```python
from build123d import *

# Parameters (mm, degrees)
BASE_FLANGE1_DEPTH = 2.3
TAB1_DEPTH         = 2.3


# Sheet-metal steps are written as plain solids
with BuildPart() as part:
    # Sketch1 → Base-Flange1 (new body)
    with BuildSketch(Plane(origin=(0, 0, 0), x_dir=(1, 0, 0), z_dir=(0, 1, 0))):
        with BuildLine():
            Line((-1, -2.15), (-2, -2.15))
            ThreePointArc((-2, -2.15), (-2.707106781, -1.857106781), (-3, -1.15))
            Line((-3, -1.15), (-3, 3.15))
            ThreePointArc((-3, 3.15), (-2.707106781, 3.857106781), (-2, 4.15))
            Line((-2, 4.15), (2, 4.15))
            ThreePointArc((2, 4.15), (2.707106781, 3.857106781), (3, 3.15))
            Line((3, 3.15), (3, -1.15))
            ThreePointArc((3, -1.15), (2.707106781, -1.857106781), (2, -2.15))
            Line((2, -2.15), (1, -2.15))
            Line((1, -2.15), (1, 2.15))
            Line((1, 2.15), (-1, 2.15))
            Line((-1, 2.15), (-1, -2.15))
        make_face()
    extrude(amount=-BASE_FLANGE1_DEPTH)

    # Sketch6 → Tab1 (add)
    with BuildSketch(Plane(origin=(0, 0, 0), x_dir=(1, 0, 0), z_dir=(0, 1, 0))):
        with BuildLine():
            Line((-1, -1.9), (-1, -1.4))
            ThreePointArc((-1, -1.4), (-0.75, -1.65), (-1, -1.9))
        make_face()
        with BuildLine():
            Line((1, -1.9), (1, -1.4))
            ThreePointArc((1, -1.4), (0.75, -1.65), (1, -1.9))
        make_face()
    extrude(amount=-TAB1_DEPTH)


solid = part.part
```
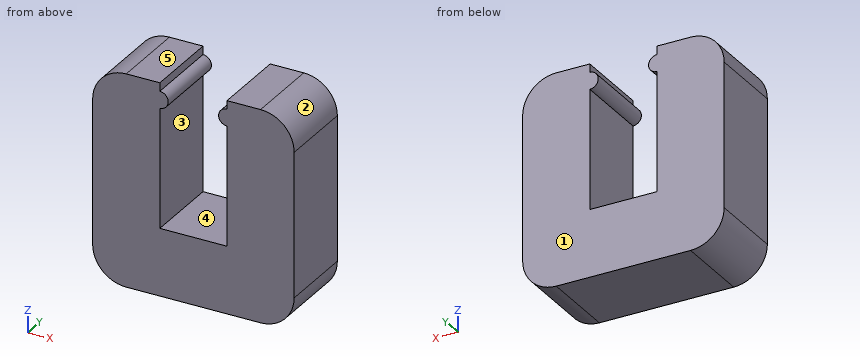
Source: CAD feature listing. Evaluate the final solid. Frame: model axes, mm. Face numbers are marked on the shaded views. A direction names the side the tool comes from. Coordinates: 2 decimals unless noted, no trailing zeros. Order: outer loops, then holes, each group sorted by start corner. A loop starts at its lowest first (then second) coordinate and runs counter-clockwise, first axis right, second up. Notation, with made-up numbers: (6, 86) - (60, 86) arc R12 ccw to (60, 102) - close; hole circle Ø6 at (-28, 14.5). An arc over 180 degrees is marked (long way). One line per item, written item: value.
1) Cut plane A-A on z = 0.5. Output: boundary loops of the cut face in (x, y), plus the area to 3 significant figures.
Computed values:
outline: (-3, -2.3) - (-1, -2.3) - (-1, 0) - (-3, 0) - close; (1, -2.3) - (3, -2.3) - (3, 0) - (1, 0) - close
area: 9.20 mm^2
2) Reachability of the marked faces 4 and 5 from +Z, -Z, +X, -X, +Y, -Y: full face, straight path, thin tool, end or side. Return the list, or none.
Computed values:
face 4: +Y, -Y
face 5: +Z, +X, -X, +Y, -Y
3) Cut plane D-D on x = -2.5. Output: boundary loops of the cut face in (y, z).
Computed values:
outline: (-2.3, -4.02) - (0, -4.02) - (0, 2.02) - (-2.3, 2.02) - close
4) Cut plane C-C on z = 1.65. Output: boundary loops of the cut face in (x, y).
Computed values:
outline: (-2.87, -2.3) - (-0.75, -2.3) - (-0.75, 0) - (-2.87, 0) - close; (0.75, -2.3) - (2.87, -2.3) - (2.87, 0) - (0.75, 0) - close
5) Ray query, line 1 (X direction, y = -1.35, z = 0); line 2 (Z direction, x = 0.4, y = -1.65); line 3 (X direction, y = -0.35, z = 1.75). Return the intervals inside material, ascending. Write a range as [from, to].
Computed values:
line 1: x = [-3, -1], [1, 3]
line 2: z = [-4.15, -2.15]
line 3: x = [-2.8, -0.77], [0.77, 2.8]
6) Mould query, pull axis Z, two halves, no side actions, for the marked faces 1, 2 and 3. Classes: released by +Z, released by -Z, zero draft, split by the parting line, or undercut.
Computed values:
face 1: zero draft
face 2: released by +Z
face 3: undercut
7) Cut plane B-B on y = -0.45. Output: boundary loops of the cut face in (x, z), plus the area to 3 significant figures.
Computed values:
outline: (-3, -3.15) arc R1 ccw to (-2, -4.15) - (2, -4.15) arc R1 ccw to (3, -3.15) - (3, 1.15) arc R1 ccw to (2, 2.15) - (1, 2.15) - (1, 1.9) arc R0.25 ccw to (1, 1.4) - (1, -2.15) - (-1, -2.15) - (-1, 1.4) arc R0.25 ccw to (-1, 1.9) - (-1, 2.15) - (-2, 2.15) arc R1 ccw to (-3, 1.15) - close
area: 28.5 mm^2
